Here's the drawing with two shaded views (mm, measured from the low corner). I have some questions. Round coordinates to 2 decimals unless told otherwise and drop trailing zeros. Write each loop counter-clockwise with the first axis right and the second up, starting at its lowest first coordinate (ties: lowest second). Pieces come first, ordered by that corner, then holes. Notation, with made-up numbers: M 72,11 L 127,11 A24 cw 127,35 Z; hole C -15.75,66.5 d1. An arc over 180 degrees is marked long. Answer as a JSON object with one key per item and string values. Group by question number.
1) Suppose I cut it at B-B, the plane z = 5.5. Write out the boundary of the cut face in (x, y) (1 decimal).
2) Please list where these lines run through material, in increasing order: L1, parallel to X at y = 2, z = 17.25 (1 decimal); L2, parallel to Z at x = 50, y = 1.3; L3, parallel to X at y = 2.15, z = 16 (1 decimal). Write a range as [from, to].
3) Suppose I cut it at A-A, the plane x = 50. Write out the boundary of the cut face in (y, z).
4) Suppose I cut it at C-C, the plane y = 2.1. Write out the boundary of the cut face in (x, z) (1 decimal), and give its area (3 significant figures).
5) I'm going to push flat-ended pins straight in: pin 1 Ø0.8 at (x, y) = (86.5, 1.5) entering from -Z (1 decimal); pin 2 Ø1.5 at (y, z) = (0.5, 10.5) entering from -X; pin 3 Ø1.3 at (y, z) = (1.5, 10) entering from +X (1 decimal). Where does each tip first touch, or does it pass through?
6) Suppose I cut it at D-D, the plane z = 15.5. State how many separate pieces and enclosed holes the cut face has, and give its area (3 significant figures).
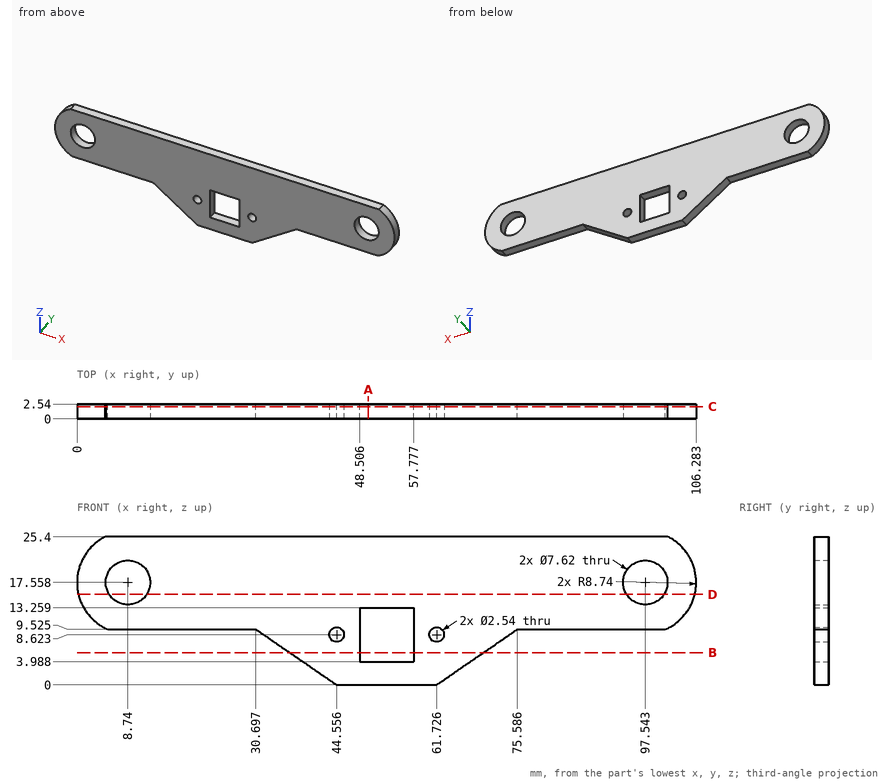
Results:
{
 "1": {"outline": "M 36.6,0 L 48.5,0 L 48.5,2.5 L 36.6,2.5 Z; M 57.8,0 L 69.7,0 L 69.7,2.5 L 57.8,2.5 Z"},
 "2": {"L1": "[0, 4.9], [12.5, 93.7], [101.3, 106.3]", "L2": "[0, 3.99], [13.26, 25.4]", "L3": "[0.1, 5.3], [12.2, 94.1], [101, 106.1]"},
 "3": {"outline": "M 0,0 L 2.54,0 L 2.54,3.99 L 0,3.99 Z; M 0,13.26 L 2.54,13.26 L 2.54,25.4 L 0,25.4 Z"},
 "4": {"outline": "M 4.9,25.4 A8.7 ccw 5.3,9.5 L 30.7,9.5 L 44.6,0 L 61.7,0 L 75.6,9.5 L 101,9.5 A8.7 ccw 101.4,25.4 Z; hole C 8.7,17.6 d7.6; hole C 44.6,8.6 d2.5; hole M 48.5,4 L 57.8,4 L 57.8,13.3 L 48.5,13.3 Z; hole C 61.7,8.6 d2.5; hole C 97.5,17.6 d7.6", "area": "1,750 mm^2"},
 "5": {"pin 1": "z = 9.5", "pin 2": "x = 2.69", "pin 3": "x = 102.9"},
 "6": {"separate pieces": "3", "enclosed holes": "0", "area": "236 mm^2"}
}
